Here's how the part is built. I have some questions about the finished solid (model axes, mm). Face numbers are marked on the shaded views. A direction names the side the tool comes from. Round coordinates to 2 decimals unless told otherwise and drop trailing zeros. Write each loop counter-clockwise with the first axis right and the second up, starting at its lowest first coordinate (ties: lowest second). Pieces come first, ordered by that corner, then holes. Notation, with made-up numbers: M 1,77.5 L 43,77.5 A31 cw 43,106.5 Z; hole C -31.75,47 d7. An arc over 180 degrees is marked long. Use a Markdown table: item, result. Add a question column.
```python
from build123d import *

# Parameters (mm, degrees)
EXTRUDE1_DEPTH     = 101.6
EXTRUDE2_DEPTH     = 1.5875
EXTRUDE3_DEPTH     = 1.5875
SKETCH4_W          = 111.125
SKETCH4_H          = 1.5875
EXTRUDE4_DEPTH     = 9.525
SKETCH5_W          = 111.125
SKETCH5_H          = 1.5875
EXTRUDE5_DEPTH     = 9.525
SKETCH6_W          = 2.431707811
SKETCH6_H          = 101.6
EXTRUDE6_DEPTH     = 25.4
SKETCH8_R          = 2.5
CUT_EXTRUDE1_DEPTH = 1.5875
CUT_EXTRUDE2_DEPTH = 3


with BuildPart() as part:
    # Sketch1 → Extrude1 (new body)
    with BuildSketch(Plane.XY):
        Polygon((101.6, 0), (101.6, 25.4), (34.925, 58.7375), (34.925, 101.6), (9.525, 101.6), (9.525, 0), (0, 0), (0, -1.5875), (11.1125, -1.5875), (11.1125, 100.0125), (33.3375, 100.0125), (33.3375, 58.7375), (100.0125, 25.4), (100.0125, -1.5875), (111.125, -1.5875), (111.125, 0), align=None)
    extrude(amount=EXTRUDE1_DEPTH)

    # Sketch2 → Extrude2 (add)
    with BuildSketch(Plane.XY.offset(101.6)):
        Polygon((0, 0), (9.525, 0), (9.525, 101.6), (34.925, 101.6), (34.925, 58.7375), (101.6, 25.4), (101.6, 0), (111.125, 0), (111.125, -1.5875), (0, -1.5875), align=None)
    extrude(amount=EXTRUDE2_DEPTH)

    # Sketch3 → Extrude3 (add)
    with BuildSketch(Plane(origin=(0, 0, 0), x_dir=(-1, 0, 0), z_dir=(0, 0, -1))):
        Polygon((-111.125, -1.5875), (-111.125, 0), (-101.6, 0), (-101.6, 25.4), (-34.925, 58.7375), (-34.925, 101.6), (-9.525, 101.6), (-9.525, 0), (0, 0), (0, -1.5875), align=None)
    extrude(amount=EXTRUDE3_DEPTH)

    # Sketch4 → Extrude4 (add)
    with BuildSketch(Plane.XY.offset(103.1875)):
        with Locations((55.5625, -0.79375)):
            Rectangle(SKETCH4_W, SKETCH4_H)
    extrude(amount=EXTRUDE4_DEPTH)

    # Sketch5 → Extrude5 (add)
    with BuildSketch(Plane(origin=(0, 0, -1.5875), x_dir=(-1, 0, 0), z_dir=(0, 0, -1))):
        with Locations((-55.5625, -0.79375)):
            Rectangle(SKETCH5_W, SKETCH5_H)
    extrude(amount=EXTRUDE5_DEPTH)

    # Sketch6 → Extrude6 (add)
    with BuildSketch(Plane(origin=(30.1625, 60.325, 0), x_dir=(0.8944271909999159, -0.44721359549995804, 0), z_dir=(-0.44721359549995804, -0.8944271909999159, 0))):
        with Locations((76.878820209, 50.8)):
            Rectangle(SKETCH6_W, SKETCH6_H)
    extrude(amount=EXTRUDE6_DEPTH)

    # Sketch8 → Cut-Extrude1 (cut)
    with BuildSketch(Plane(origin=(69.85, -34.925, 0), x_dir=(0, 0, -1), z_dir=(0.8944271909999159, -0.447213595499958, 0))):
        with Locations(Location((-50.8, 51.635400371, 0), (0, 0, 90))):
            Circle(SKETCH8_R)
    extrude(amount=-CUT_EXTRUDE1_DEPTH, mode=Mode.SUBTRACT)

    # Sketch9 → Cut-Extrude2 (cut)
    with BuildSketch(Plane(origin=(30.48, 60.96, 0), x_dir=(-0.8944271909999159, 0.44721359549995804, 0), z_dir=(0.44721359549995804, 0.8944271909999159, 0))):
        with BuildLine():
            Line((-25.4, 44.45), (-11.1125, 44.45))
            ThreePointArc((-11.1125, 44.45), (-8.86743597, 43.52006403), (-7.9375, 41.275))
            Line((-7.9375, 41.275), (-7.9375, 12.7))
            ThreePointArc((-7.9375, 12.7), (-8.86743597, 10.45493597), (-11.1125, 9.525))
            Line((-11.1125, 9.525), (-25.4, 9.525))
            ThreePointArc((-25.4, 9.525), (-27.64506403, 10.45493597), (-28.575, 12.7))
            Line((-28.575, 12.7), (-28.575, 41.275))
            ThreePointArc((-28.575, 41.275), (-27.64506403, 43.52006403), (-25.4, 44.45))
        make_face()
    extrude(amount=-CUT_EXTRUDE2_DEPTH, mode=Mode.SUBTRACT)


solid = part.part
```
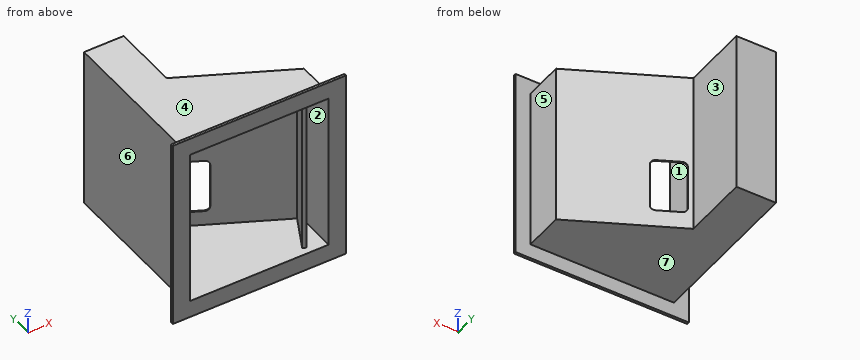
Item 1: Imagine slicing it at C-C on z = 57. List the corners of the cut face in (x, y) for me (1 decimal).
Item 2: If we mould it in two halves opening along Z, with no side actions, what happens to the marked faces 1, 2, 3 and 4? For each: +Z half, -Z half, draft (parallel to the pull), parting line (faces both ways), or undercut.
Item 3: I need wall thicknesses on probe 1 along Z at (x, y) = (67, 16); probe 2 along X at (y, z) = (65, 1.5) (1 decimal); probe 3 along X at (y, z) = (9, 87) (1 decimal). Which ranges of each line are inside material? Lowest first, please. Write a range as from..to.
Item 4: Imagine slicing it at D-D on x = 24. List the corners of the cut face in (y, z) for me, plus the area to 3 significant figures.
Item 5: For pin 1 Ø18 at (x, z) = (21, 31) entering from -Y; pin 2 Ø3 at (x, y) = (21.5, 73) entering from -Z; pin 3 Ø5 at (x, z) = (67.5, 21) entering from +Y, each with a flat end and sliding along its axis, tell me the tip position at first contact or that it passes through.
Item 6: Imagine slicing it at A-A on z = 27. List the corners of the cut face in (x, y) for me (1 decimal).
Item 7: Imagine slicing it at B-B on y = 73. List the corners of the cut face in (x, z) for me (1 decimal), plus the area to 3 significant figures.
Item 8: On a 3-axis mill with a long thin cutter (end or side, diameter ignored), from which of +Z, -Z, +X, -X, +Y, -Y can I reach the whole of each face in a straight line? I mean the marked faces 5, 6 and 7. Say none if no direction works.
The answers:
| question | item | result |
|---|---|---|
| 1 | outline | M 0,-1.6 L 11.1,-1.6 L 11.1,100 L 33.3,100 L 33.3,58.7 L 97.8,26.5 L 86.5,3.8 L 88.7,2.7 L 100,25.4 L 100,-1.6 L 111.1,-1.6 L 111.1,0 L 101.6,0 L 101.6,25.4 L 34.9,58.7 L 34.9,101.6 L 9.5,101.6 L 9.5,0 L 0,0 Z |
| 2 | face 1 | undercut |
| 2 | face 2 | undercut |
| 2 | face 3 | draft |
| 2 | face 4 | +Z half |
| 3 | probe 1 | -1.59..0, 101.6..103.19 |
| 3 | probe 2 | 9.5..11.1, 33.3..34.9 |
| 3 | probe 3 | 9.5..11.1, 89.1..91.8, 100..101.6 |
| 4 | outline | M -1.59,-11.11 L 0,-11.11 L 0,-1.59 L 101.6,-1.59 L 101.6,103.19 L 0,103.19 L 0,112.71 L -1.59,112.71 L -1.59,101.6 L 100.01,101.6 L 100.01,0 L -1.59,0 Z |
| 4 | area | 519 mm² |
| 5 | pin 1 | y = 100.01 |
| 5 | pin 2 | z = -1.59 |
| 5 | pin 3 | y = 43.7 |
| 6 | outline | M 0,-1.6 L 11.1,-1.6 L 11.1,100 L 33.3,100 L 33.3,58.7 L 37.3,56.8 L 37.6,57.4 L 34.9,58.7 L 34.9,101.6 L 9.5,101.6 L 9.5,0 L 0,0 Z; M 55.7,47.5 L 97.8,26.5 L 86.5,3.8 L 88.7,2.7 L 100,25.4 L 100,-1.6 L 111.1,-1.6 L 111.1,0 L 101.6,0 L 101.6,25.4 L 56,48.2 Z |
| 7 | outline | M 9.5,-1.6 L 34.9,-1.6 L 34.9,103.2 L 9.5,103.2 Z; hole M 11.1,0 L 33.3,0 L 33.3,101.6 L 11.1,101.6 Z |
| 7 | area | 403 mm² |
| 8 | face 5 | +Z, -Z, +X, +Y |
| 8 | face 6 | +Z, -Z, -X, +Y |
| 8 | face 7 | -Z, +X, -X, +Y |
